Here's how the part is built. I have some questions about the finished solid (model axes, mm). A direction names the side the tool comes from. Coordinates: 2 decimals unless noted, no trailing zeros. Write each loop counter-clockwise with the first axis right and the second up, starting at its lowest first coordinate (ties: lowest second). Pieces come first, ordered by that corner, then holes. Notation, with made-up numbers: (50.5, 41) -> (68.5, 41) arc R7 ccw to (68.5, 51) -> close; hole circle Ø6 at (-5.5, -19.75). An arc over 180 degrees is marked (long way). Put each result on its own line as item: value.
Solid Edge part; units mm, degrees
sketch "Sketch1" plane through (0, 0, 0) normal (0, -1, 0) x (1, 0, 0)
  line L0 (-20, -2.5) -> (20, -2.5)
  line L1 (20, -2.5) -> (20, 2.5)
  line L2 (20, 2.5) -> (-20, 2.5)
  line L3 (-20, 2.5) -> (-20, -2.5)
  dimension "D1" = 20
  dimension "D2" = 20
extrude "Protrusion1" add sketch "Sketch1" against normal blind 60
sketch "Sketch2" plane through (20, 30, 0) normal (1, 0, 0) x (0, 1, 0)
  line L0 (-9, 2.5) -> (9, 2.5)
  line L1 (9, 2.5) -> (9, 2.3)
  line L2 (9, 2.3) -> (-9, 2.3)
  line L3 (-9, 2.3) -> (-9, 2.5)
  dimension "D1" = 9
  dimension "D2" = 9
extrude "Cutout1" cut sketch "Sketch2" against normal through all
sketch "Sketch3" plane through (0, 49.5, 2.5) normal (0, 0, 1) x (1, 0, 0)
  circle A0 centre (0, -19.5) radius 2.5
extrude "Cutout2" cut sketch "Sketch3" against normal through all
chamfer "Fase_1" distance 0.7 angle 45 2 edges at (0, 32.5, 2.3) (2.5, 30, -2.5)
properties material "Nylon, allgemein"
Item 1: Imagine slicing it at A-A on x = 0. Write out the boundary of the cut face in (y, z), then the cut area to 3 significant figures.
Output:
outline: (0, -2.5) -> (26.8, -2.5) -> (27.5, -1.8) -> (27.5, 1.6) -> (26.8, 2.3) -> (21, 2.3) -> (21, 2.5) -> (0, 2.5) -> close; (32.5, -1.8) -> (33.2, -2.5) -> (60, -2.5) -> (60, 2.5) -> (39, 2.5) -> (39, 2.3) -> (33.2, 2.3) -> (32.5, 1.6) -> close
area: 271 mm²
Item 2: For P1, Ø1.5, axis at x = 3.5, z = -1.5, coming from the -Y side; P2, Ø6.5, axis at x = 0, y = 30, coming from the +Z side, each with a flat end and sliding along its axis, tell me the tip position at first contact or that it passes through.
Output:
P1: stops at y = 0
P2: stops at z = 2.3
Item 3: Imagine slicing it at B-B on y = 30. Write out the boundary of the cut face in (x, z).
Output:
outline: (-20, -2.5) -> (-3.2, -2.5) -> (-2.5, -1.8) -> (-2.5, 1.6) -> (-3.2, 2.3) -> (-20, 2.3) -> close; (2.5, -1.8) -> (3.2, -2.5) -> (20, -2.5) -> (20, 2.3) -> (3.2, 2.3) -> (2.5, 1.6) -> close
Item 4: If we mould it in two halves opening along X, with no side actions, what happens to faces 1 (the flat face through (20, 30, 0)), 2 (the cylindrical face through (1.34, 32.11, -0.08)), 3 (the flat face through (4, 30, -2.5)), 4 (the flat face through (-20, 30, 0))? For each: released by +X, released by -X, zero draft, split by the parting line, or undercut.
Output:
face 1: released by +X
face 2: undercut
face 3: zero draft
face 4: released by -X
Item 5: Which directions (+Z, -Z, +X, -X, +Y, -Y) give clear straight access to the entire face, cutting with the end or side of a thin tool? Please do faces 5 (the flat face through (0, 34, 2.3)), 6 (the flat face through (0, 0, 0)).
Output:
face 5: +Z, +X, -X
face 6: +Z, -Z, +X, -X, -Y
Item 6: Imagine slicing it at C-C on y = 22. Write out the boundary of the cut face in (x, z), then the cut area to 3 significant figures.
Output:
outline: (-20, -2.5) -> (20, -2.5) -> (20, 2.3) -> (-20, 2.3) -> close
area: 192 mm²
Item 7: Please list where these lines run through material, in increasing order: line 1 along Y through (x, z) = (0, -0.3); line 2 along Z through (x, y) = (-6, 23.5). Write a range as from..to.
Output:
line 1: y = 0..27.5, 32.5..60
line 2: z = -2.5..2.3
